Input: part model. Units: mm. Frame: model coordinates. A direction names the side the tool comes from. Round coordinates to 2 decimals unless told otherwise and drop trailing zeros. Loops run counter-clockwise (first coordinate to the right, second up) from the corner with the lowest first, then second, coordinate; pieces in that order, holes last. Notation, with made-up numbers: M 33.5,83 L 66.5,83 A19 ccw 66.5,117 Z; hole C 82.5,61 d2. An arc over 180 degrees is marked long. Return JSON: item names as keys, results as strings. Group by question number.
1) Mould query, pull axis Z, two halves, no side actions, for faces 1 (the face through (-91, 21, 0)), 2 (the face through (-64.4, 42.3, -10)), 3 (the face through (-105.315, 8.504, -0.596)). Classes: +Z half, -Z half, draft (parallel to the pull), parting line (faces both ways), or undercut.
2) Section D-D (y = 9). Output: boundary loops of the cut face in (x, z).
3) Material intervals for line 1 (X direction, y = 55.25, z = 0); line 2 (X direction, y = 12.75, z = 0); line 3 (Z direction, x = -62, y = 52), sorted ascending. Write a range as from..to.
4) Contact query for flat-ended pins moving along their axis: P1, Ø5, axis at x = -22, z = 0, coming from the +Y side; P2, Ø7, axis at x = -62, z = 0, coming from the -Y side; P3, Ø6, axis at x = -105.5, z = 3.5, coming from the +Y side; P4, Ø1, axis at y = 23.5, z = 5.5, coming from the +X side. Output: stop coordinate, or through.
5) Section A-A (z = 0). Count the separate pieces of the cut face and the enclosed holes in it, plus the area to 3 significant figures.
6) Access query for faces 4 (the face through (-127, 7, 0)), 5 (the face through (-111, 20, -5)), 6 (the face through (-74, 19, 0)). Directions: +Z, -Z, +X, -X, +Y, -Y. A direction counts if a zero-diameter tool reaches every point of the face in a straight line with its end or side. Return the directions, or none.
7) Section C-C (y = 54). Output: boundary loops of the cut face in (x, z).
8) Section B-B (x = -62). Output: boundary loops of the cut face in (y, z).
Autodesk Inventor part; units mm, degrees
ref_plane "YZ Plane" through (0, 0, 0) normal (1, 0, 0) x (0, 1, 0)
ref_plane "XZ Plane" through (0, 0, 0) normal (0, 1, 0) x (-1, 0, 0)
ref_plane "XY Plane" through (0, 0, 0) normal (0, 0, 1) x (1, 0, 0)
sketch "Sketch1" plane through (0, 0, 0) normal (0, 0, 1) x (1, 0, 0)
  line L0 (-89, 58) -> (0, 58)
  line L1 (0, 42) -> (-74, 42)
  line L2 (-74, 42) -> (-74, 0)
  line L3 (-74, 0) -> (-127, 0)
  line L4 (-127, 0) -> (-127, 20)
  line L5 (-127, 20) -> (-89, 20)
  line L6 (-89, 20) -> (-89, 58)
  line L7 (0, 58) -> (0, 42)
  point P0 (0, 0)
  point P1 (0, 50)
  point P2 (-100.5, 0)
  dimension "d116" = 15
  dimension "d128" = 89
  dimension "d129" = 16
  dimension "d130" = 20
  dimension "d131" = 53
  dimension "d132" = 38
  dimension "d135" = 74
extrude "Soporte" add sketch "Sketch1" along normal mid plane 20
sketch "Sketch13" plane through (-74, 42, 10) normal (0, 1, 0) x (1, 0, 0)
  line L0 (12, 10) -> (52, 10) construction
  line L1 (0, 20) -> (0, 0)
  line L2 (0, 0) -> (74, 0)
  point P0 (74, 10)
  point P1 (32, 10)
  point P2 (-15, 20)
  point P3 (74, 20)
  point P4 (0, 10)
  dimension "d104" = 40
  dimension "d133" = 32
hole "BCA M5" at (-62, 42, 0) at (-22, 42, 0) direction (0, 1, 0) diameter 5.5 end through all countersink diameter 11 countersink angle 90
fillet "Fillet7" radius 5 4 edges at (-89, 20, 0) (-74, 42, 0) (-127, 20, 0) (0, 42, 0)
sketch "Sketch15" plane through (-122, 20, 10) normal (0, 1, 0) x (1, 0, 0)
  line L0 (28, 0) -> (0, 0)
  line L1 (0, 0) -> (0, 20)
  point P0 (122, 10)
  point P1 (14, 10)
  point P2 (14, 0)
  point P3 (0, 10)
hole "Hole8" at (-108, 20, 0) direction (0, -1, 0) diameter 5.5 end through all countersink diameter 11 countersink angle 90
properties part number "unión placa soporte TIC DC" material "PET Plastic"
Returned:
{
 "1": {"face 1": "draft", "face 2": "-Z half", "face 3": "undercut"},
 "2": {"outline": "M -127,-10 L -74,-10 L -74,10 L -127,10 Z; hole C -108,0 d5.5"},
 "3": {"line 1": "x = -89..-64.75, -59.25..-24.75, -19.25..0", "line 2": "x = -127..-110.75, -105.25..-74", "line 3": "z = -10..-2.75, 2.75..10"},
 "4": {"P1": "passes through", "P2": "stops at y = 44", "P3": "stops at y = 20", "P4": "stops at x = -74"},
 "5": {"separate pieces": "4", "enclosed holes": "0", "area": "2,510 mm^2"},
 "6": {"face 4": "+Z, -Z, -X, +Y, -Y", "face 5": "+Z, -Z, -X, +Y", "face 6": "+Z, -Z, +X, -Y"},
 "7": {"outline": "M -89,-10 L 0,-10 L 0,10 L -89,10 Z; hole C -62,0 d5.5; hole C -22,0 d5.5"},
 "8": {"outline": "M 42,-10 L 58,-10 L 58,-2.75 L 44.75,-2.75 L 42,-5.5 Z; M 42,5.5 L 44.75,2.75 L 58,2.75 L 58,10 L 42,10 Z"}
}
